Build history of the part. All positions in model axes, mm. A direction names the side the tool comes from. Round coordinates to 2 decimals unless told otherwise and drop trailing zeros. Write each loop counter-clockwise with the first axis right and the second up, starting at its lowest first coordinate (ties: lowest second). Pieces come first, ordered by that corner, then holes. Notation, with made-up numbers: (24, 53) -> (64, 53) arc R26 cw to (64, 87) -> close; hole circle Ø9 at (21.5, 49). An arc over 180 degrees is marked (long way). Answer in a Markdown table with one row per item. Add a question column.
from build123d import *

# Parameters (mm, degrees)
F1_DEPTH = 20.32


# Not quite as in the source:
# - the arcs of a loft's sections are written as splines that run evenly, so that the points pair up as in the source's solid
# - a feature names something its author has since deleted; it is built from what else it names


with BuildPart() as f1:
    # F0 (on Top) → F1 (new body)
    with BuildSketch(Plane.XY):
        with BuildLine():
            ThreePointArc((0, -31.75), (31.75, 0), (0, 31.75))
            Line((0, 31.75), (0, -31.75))
        make_face()
    extrude(amount=F1_DEPTH)

    # F4 (on offset) → F6 section 0
    with BuildSketch(Plane.XY.offset(20.32)):
        with BuildLine():
            add(Edge.make_bspline(
                [(0, 31.7974612136), (-1.8499013065, 31.7974612136), (-3.6997740452, 31.63561832), (-7.3433683431, 30.9931543385), (-9.1370336348, 30.5125431721), (-12.6137108486, 29.2471361521), (-14.2966690809, 28.4623598401), (-17.5007921327, 26.6124585335), (-19.0219074714, 25.5473621069), (-21.8561207037, 23.169174829), (-23.169174829, 21.8561207037), (-25.5473621069, 19.0219074714), (-26.6124585335, 17.5007921327), (-27.5374091868, 15.8987306068)],
                knots=[0, 0, 0, 0, 0.1666666667, 0.1666666667, 0.3333333333, 0.3333333333, 0.5, 0.5, 0.6666666667, 0.6666666667, 0.8333333333, 0.8333333333, 1, 1, 1, 1], degree=3))
            add(Edge.make_bspline(
                [(-27.5374091868, 15.8987306068), (-28.4623598401, 14.2966690809), (-29.2471361521, 12.6137108486), (-30.5125431721, 9.1370336348), (-30.9931543385, 7.3433683431), (-31.63561832, 3.6997740452), (-31.7974612136, 1.8499013065), (-31.7974612136, -1.8499013065), (-31.63561832, -3.6997740452), (-30.9931543385, -7.3433683431), (-30.5125431721, -9.1370336348), (-29.2471361521, -12.6137108486), (-28.4623598401, -14.2966690809), (-27.5374091868, -15.8987306068)],
                knots=[0, 0, 0, 0, 0.1666666667, 0.1666666667, 0.3333333333, 0.3333333333, 0.5, 0.5, 0.6666666667, 0.6666666667, 0.8333333333, 0.8333333333, 1, 1, 1, 1], degree=3))
            add(Edge.make_bspline(
                [(-27.5374091868, -15.8987306068), (-26.6124585335, -17.5007921327), (-25.5473621069, -19.0219074714), (-23.169174829, -21.8561207037), (-21.8561207037, -23.169174829), (-19.0219074714, -25.5473621069), (-17.5007921327, -26.6124585335), (-14.2966690809, -28.4623598401), (-12.6137108486, -29.2471361521), (-9.1370336348, -30.5125431721), (-7.3433683431, -30.9931543385), (-3.6997740452, -31.63561832), (-1.8499013065, -31.7974612136), (0, -31.7974612136)],
                knots=[0, 0, 0, 0, 0.1666666667, 0.1666666667, 0.3333333333, 0.3333333333, 0.5, 0.5, 0.6666666667, 0.6666666667, 0.8333333333, 0.8333333333, 1, 1, 1, 1], degree=3))
            add(Edge.make_bspline(
                [(0, -31.7974612136), (1.8499013065, -31.7974612136), (3.6997740452, -31.63561832), (7.3433683431, -30.9931543385), (9.1370336348, -30.5125431721), (12.6137108486, -29.2471361521), (14.2966690809, -28.4623598401), (17.5007921327, -26.6124585335), (19.0219074714, -25.5473621069), (21.8561207037, -23.169174829), (23.169174829, -21.8561207037), (25.5473621069, -19.0219074714), (26.6124585335, -17.5007921327), (27.5374091868, -15.8987306068)],
                knots=[0, 0, 0, 0, 0.1666666667, 0.1666666667, 0.3333333333, 0.3333333333, 0.5, 0.5, 0.6666666667, 0.6666666667, 0.8333333333, 0.8333333333, 1, 1, 1, 1], degree=3))
            add(Edge.make_bspline(
                [(27.5374091868, -15.8987306068), (28.4623598401, -14.2966690809), (29.2471361521, -12.6137108486), (30.5125431721, -9.1370336348), (30.9931543385, -7.3433683431), (31.63561832, -3.6997740452), (31.7974612136, -1.8499013065), (31.7974612136, 1.8499013065), (31.63561832, 3.6997740452), (30.9931543385, 7.3433683431), (30.5125431721, 9.1370336348), (29.2471361521, 12.6137108486), (28.4623598401, 14.2966690809), (27.5374091868, 15.8987306068)],
                knots=[0, 0, 0, 0, 0.1666666667, 0.1666666667, 0.3333333333, 0.3333333333, 0.5, 0.5, 0.6666666667, 0.6666666667, 0.8333333333, 0.8333333333, 1, 1, 1, 1], degree=3))
            add(Edge.make_bspline(
                [(27.5374091868, 15.8987306068), (26.6124585335, 17.5007921327), (25.5473621069, 19.0219074714), (23.169174829, 21.8561207037), (21.8561207037, 23.169174829), (19.0219074714, 25.5473621069), (17.5007921327, 26.6124585335), (14.2966690809, 28.4623598401), (12.6137108486, 29.2471361521), (9.1370336348, 30.5125431721), (7.3433683431, 30.9931543385), (3.6997740452, 31.63561832), (1.8499013065, 31.7974612136), (0, 31.7974612136)],
                knots=[0, 0, 0, 0, 0.1666666667, 0.1666666667, 0.3333333333, 0.3333333333, 0.5, 0.5, 0.6666666667, 0.6666666667, 0.8333333333, 0.8333333333, 1, 1, 1, 1], degree=3))
        make_face()
    # F5 (on offset) → F6 section 1
    with BuildSketch(Plane.XY.offset(50.8)):
        Polygon((27.536238076, 15.8980544657), (0, 31.7961089313), (-27.536238076, 15.8980544657), (-27.536238076, -15.8980544657), (0, -31.7961089313), (27.536238076, -15.8980544657), align=None)
    loft(ruled=True)


solid = f1.part
(1) Drop flat-ended pins along their axis: P1, Ø5, axis at y = 12.5, z = 22.5, coming from the +X side; P2, Ø10, axis at y = 21, z = 11, coming from the +X side; P3, Ø3, axis at y = 6.5, z = 13.5, coming from the -X side. Give the stop position or say it passes through.
(2) Which spindle directions (+Z, -Z, +X, -X, +Y, -Y) get a long thin tool onto all of the face, cutting with end or side? Do faces 1 (the face through (0, 0, 10)), 2 (the face through (12, 0, 0)). Say none if no direction does.
(3) Saw through at A-A (z = 4.5). List the corners of the cut face in (x, y).
(4) Probe line 1 along Z through (x, y) = (-3, 3.5); line 2 along X through (y, z) = (8, 25); line 3 along Y through (x, z) = (-1, 37.5). List the from-to ranges inside material, lowest first.
Answer sheet:
| question | item | result |
|---|---|---|
| 1 | P1 | stops at x = 30.02 |
| 1 | P2 | stops at x = 27.42 |
| 1 | P3 | stops at x = 0 |
| 2 | face 1 | -Z, -X, +Y, -Y |
| 2 | face 2 | -Z, +X, -X, +Y, -Y |
| 3 | outline | (0, -31.75) arc R31.75 ccw to (0, 31.75) -> close |
| 4 | line 1 | z = 20.32 to 50.8 |
| 4 | line 2 | x = -30.27 to 30.27 |
| 4 | line 3 | y = -31.49 to 31.49 |
